```python
from build123d import *

# Parameters (mm, degrees)
BOSS_EXTRUDE1_DEPTH     = 105
SKETCH2_W               = 20.5
SKETCH2_H               = 3
CUT_EXTRUDE1_DEPTH      = 1
CUT_EXTRUDE1_DEPTH_BACK = 106


with BuildPart() as part:
    # Sketch1 → Boss-Extrude1 (new body)
    with BuildSketch(Plane.XY):
        Polygon((18, 11.742640687), (13.25, 16.492640687), (13.25, 38.25), (-13.25, 38.25), (-13.25, 16.492640687), (-18, 11.742640687), (-18, -3), (18, -3), align=None)
        Polygon((15, 0), (-15, 0), (-15, 10.5), (-10.25, 15.25), (-10.25, 35.25), (10.25, 35.25), (10.25, 15.25), (15, 10.5), align=None, mode=Mode.SUBTRACT)
    extrude(amount=BOSS_EXTRUDE1_DEPTH)

    # Sketch2 → Cut-Extrude1 (cut, two sides)
    with BuildSketch(Plane.XY.offset(105)) as cut_extrude1_sk:
        with Locations((0, 36.75)):
            Rectangle(SKETCH2_W, SKETCH2_H)
    extrude(amount=CUT_EXTRUDE1_DEPTH, mode=Mode.SUBTRACT)
    extrude(cut_extrude1_sk.sketch, amount=-CUT_EXTRUDE1_DEPTH_BACK, mode=Mode.SUBTRACT)


solid = part.part
```
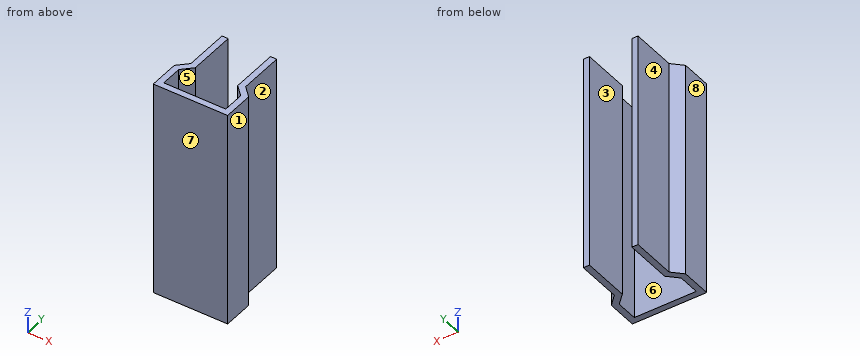
Input: part model. Units: mm. Frame: model coordinates. Face numbers are marked on the shaded views. A direction names the side the tool comes from. Give positions to 0.01 mm unless a question says otherwise; leave off trailing zeros. Order: outer loops, then holes, each group sorted by start corner. A loop starts at its lowest first (then second) coordinate and runs counter-clockwise, first axis right, second up. Notation, with made-up numbers: (13, 77.25) - (23, 77.25) arc R22 ccw to (23, 86.25) - close; hole circle Ø3 at (87.5, 79.5). An arc over 180 degrees is marked (long way). Use a Markdown table: item, result.
(1) Line query: line 1 (X direction, y = 1.5, z = 43.5); line 2 (X direction, y = 19.5, z = 81); line 3 (Y direction, x = -4, z = 13). Output: solid intervals per line, ascending. Write a range as from..to.
Computed values:
| item | result |
|---|---|
| line 1 | x = -18..-15, 15..18 |
| line 2 | x = -13.25..-10.25, 10.25..13.25 |
| line 3 | y = -3..0 |
(2) Section query C-C (x = 3.5). Output: boundary loops of the cut face in (y, z).
Computed values:
| item | result |
|---|---|
| outline | (-3, 0) - (0, 0) - (0, 105) - (-3, 105) - close |
(3) Section query A-A (y = 5.5). Output: boundary loops of the cut face in (x, z).
Computed values:
| item | result |
|---|---|
| outline | (-18, 0) - (-15, 0) - (-15, 105) - (-18, 105) - close; (15, 0) - (18, 0) - (18, 105) - (15, 105) - close |
(4) Pin query (flat end, axial travel): pin 1 (11 mm diameter, centred on y = 26, z = 71.5, fed in from -X); pin 2 (1.5 mm diameter, centred on x = 13.5, y = 2.5, fed in from -Z); pin 3 (24 mm diameter, centred on y = 26, z = 55, fed in from +X); pin 4 (7 mm diameter, centred on y = 29, z = 69.5, fed in from +X). Return the tip coordinate at first contact, or that it passes through.
Computed values:
| item | result |
|---|---|
| pin 1 | stops at x = -13.25 |
| pin 2 | passes through |
| pin 3 | stops at x = 15.74 |
| pin 4 | stops at x = 13.25 |
(5) Access query for the marked faces 1, 2, 3, 4 and 5. Directions: +Z, -Z, +X, -X, +Y, -Y. A direction counts if a zero-diameter tool reaches every point of the face in a straight line with its end or side. Return the directions, or none.
Computed values:
| item | result |
|---|---|
| face 1 | +Z, -Z, +X, +Y, -Y |
| face 2 | +Z, -Z, +X, +Y |
| face 3 | +Z, -Z, +Y |
| face 4 | +Z, -Z, -X, +Y |
| face 5 | +Z, -Z |
(6) Section query B-B (z = 32). Output: boundary loops of the cut face in (x, y).
Computed values:
| item | result |
|---|---|
| outline | (-18, -3) - (18, -3) - (18, 11.74) - (13.25, 16.49) - (13.25, 38.25) - (10.25, 38.25) - (10.25, 15.25) - (15, 10.5) - (15, 0) - (-15, 0) - (-15, 10.5) - (-10.25, 15.25) - (-10.25, 38.25) - (-13.25, 38.25) - (-13.25, 16.49) - (-18, 11.74) - close |
(7) Draft query along X for the marked faces 6, 7 and 8. Return one class per face: released by +X, released by -X, zero draft, split by the parting line, or undercut.
Computed values:
| item | result |
|---|---|
| face 6 | undercut |
| face 7 | zero draft |
| face 8 | released by -X |
(8) Section query D-D (y = 14). Output: boundary loops of the cut face in (x, z), then the cut area to 3 significant figures.
Computed values:
| item | result |
|---|---|
| outline | (-15.74, 0) - (-11.5, 0) - (-11.5, 105) - (-15.74, 105) - close; (11.5, 0) - (15.74, 0) - (15.74, 105) - (11.5, 105) - close |
| area | 891 mm2 |
